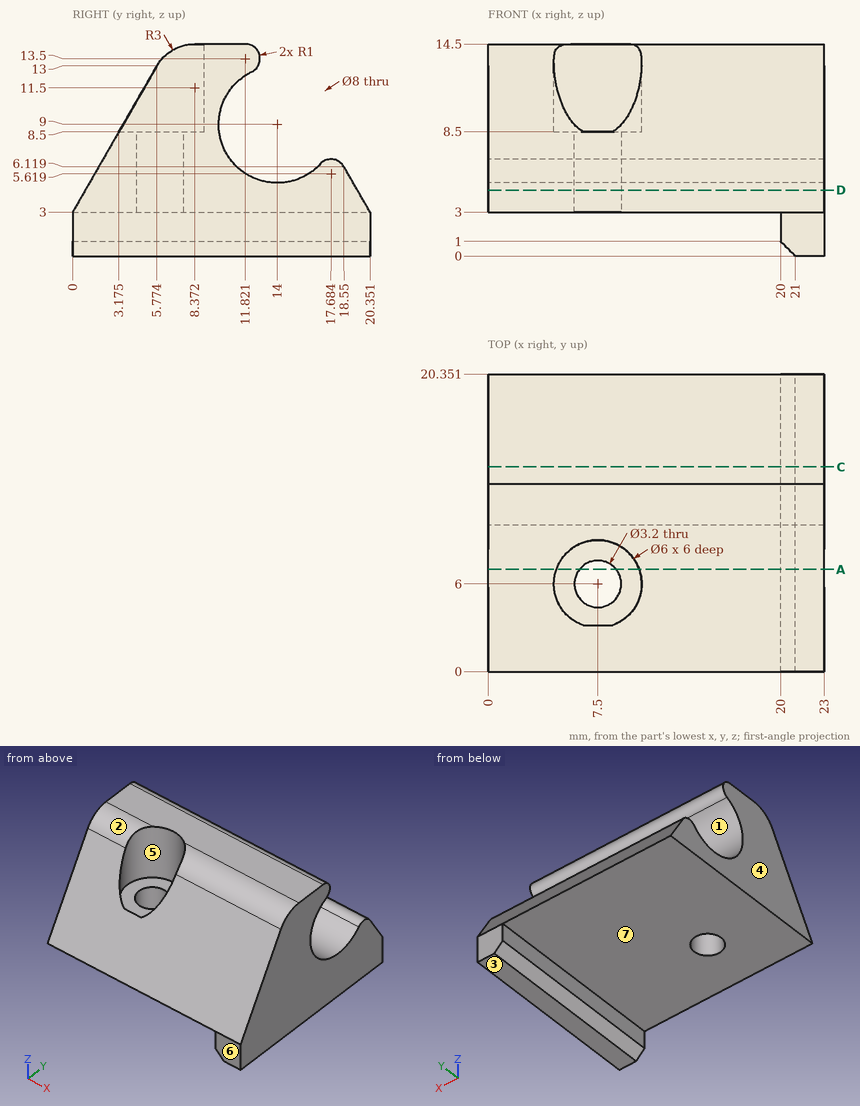
Check sheet for the drawn part. Datum: minimum x, y, z corner. Units: mm. A direction names the side the tool comes from. Round coordinates to 2 decimals unless told otherwise and drop trailing zeros. Order: outer loops, then holes, each group sorted by start corner. A loop starts at its lowest first (then second) coordinate and runs counter-clockwise, first axis right, second up. Notation, with made-up numbers: (80.5, 66.5) -> (103.5, 66.5) arc R19 cw to (103.5, 96.5) -> close; hole circle Ø7 at (-22, 89.5). An arc over 180 degrees is marked (long way). Put each result on its own line as item: value. Start each with the question number.
(1) Material ranges on line 1 along X through (y, z) = (6, 13.25); line 2 along Y through (x, z) = (7, 4.25); line 3 along Z through (x, y) = (16, 11) (1 decimal), recorded low to high.
(2) Draft check along Z on the marked faces 1, 2, 3 and 4. Enter one of: +Z half, -Z half, draft (parallel to the pull), parting line (faces both ways), or undercut.
(3) Tool access check on the marked faces 5, 6 and 7. Record the directions out of +Z, -Z, +X, -X, +Y, -Y that give a thin tool (end or side, any length) a straight path to the whole face; none if there is none.
(4) Section check A-A (y = 7). Enter the section's corners in (x, z).
(5) Section check D-D (z = 4.5). Enter the section's corners in (x, y) (1 decimal).
(6) Section check C-C (y = 14). Enter the section's corners in (x, z).
(7) Depth check by flat-ended pin: pin 1 Ø1 at (y, z) = (9.5, 1.5) entering from -X; pin 2 Ø1 at (x, y) = (20, 15) entering from -Z; pin 3 Ø5.5 at (x, y) = (7.5, 6) entering from -Z. Enter the tip coordinate at first touch or a pass-through.
Completed:
1. line 1: x = 0 to 4.5, 10.5 to 23
1. line 2: y = 0.72 to 4.48, 7.52 to 19.63
1. line 3: z = 3 to 6.4, 11.6 to 14.5
2. face 1: undercut
2. face 2: +Z half
2. face 3: -Z half
2. face 4: draft
3. face 5: +Z
3. face 6: +Z, -Z, +X, -X, -Y
3. face 7: -Z, -X, +Y, -Y
4. outline: (0, 3) -> (6.25, 3) -> (6.25, 8.5) -> (4.67, 8.5) -> (4.67, 14.17) -> (0, 14.17) -> close; (8.75, 3) -> (20, 3) -> (20, 1) -> (21, 0) -> (23, 0) -> (23, 14.17) -> (10.33, 14.17) -> (10.33, 8.5) -> (8.75, 8.5) -> close
5. outline: (0, 0.9) -> (23, 0.9) -> (23, 19.5) -> (0, 19.5) -> close; hole circle Ø3.2 at (7.5, 6)
6. outline: (0, 3) -> (20, 3) -> (20, 1) -> (21, 0) -> (23, 0) -> (23, 5) -> (0, 5) -> close
7. pin 1: stops at x = 20
7. pin 2: stops at z = 0.5
7. pin 3: stops at z = 3
